The listing builds one solid part. Answer for the finished solid, in the listing's coordinates (mm). Face numbers are marked on the shaded views. A direction names the side the tool comes from. Coordinates: 2 decimals unless noted, no trailing zeros. Order: outer loops, then holes, each group sorted by start corner. A loop starts at its lowest first (then second) coordinate and runs counter-clockwise, first axis right, second up. Notation, with made-up numbers: (75.5, 1) - (112.5, 1) arc R25 ccw to (112.5, 35) - close; hole circle Ø5 at (-12, -5.75). An arc over 180 degrees is marked (long way). Use a Markdown table: item, result. Add a question column.
Item 1: For the marked faces 1 and 2, determine the directions among +Z, -Z, +X, -X, +Y, -Y from which every point of the face is accessible in a straight line to the end or side of a thin tool.
Item 2: The part is cut by section C-C, the plane z = 14.25. State how many separate pieces and enclosed holes the cut face has, then the cut area to 3 significant figures.
Item 3: Flat-ended cylindrical pins translate along their axes: P1, Ø12.5, axis at x = -11, y = 16, coming from the +Z side; P2, Ø12, axis at x = 22.5, y = 22.5, coming from the +Z side. Find the tip coordinate at first contact, or state that the pin passes through.
Item 4: The mould has two halves that part along Y. Classify the marked faces 3, 4, 5 and 6: released by +Y, released by -Y, zero draft, split by the parting line, or undercut.
Item 5: The part is cut by section B-B, the plane y = -19.5. Give the vertices of the cut face in (x, z) (3 decimals), then the cut area to 3 significant figures.
Item 6: The part is cut by section D-D, the plane y = 5. Give the vertices of the cut face in (x, z) (3 decimals), then the cut area to 3 significant figures.
Item 7: The part is cut by section A-A, the plane x = 31.5. Give the vertices of the cut face in (y, z) (3 decimals).
Item 8: Find the intervals of material crossed by line 1 along X through (y, z) = (3, 15.75) (3 decimals); line 2 along Y through (x, z) = (-29.5, 3.25) (3 decimals); line 3 along Y through (x, z) = (-11, 9.5) (3 decimals), in increasing order.
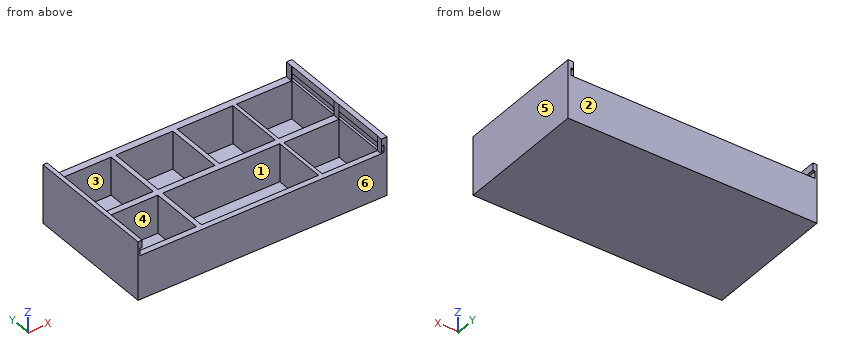
from build123d import *

# Parameters (mm, degrees)
F0_W      = 107.95
F0_H      = 57.15
F1_DEPTH  = 25.4
F2_W      = 25.4
F2_H      = 25.4
F2_H_2    = 23.2541756704
F2_W_2    = 24.6955640614
F2_W_3    = 50.8
F2_H_3    = 23.3953045681
F2_W_4    = 24.2106489923
F2_W_5    = 24.0074023604
F2_H_4    = 23.0993351433
F3_DEPTH  = 22.86
F4_W      = 103.6651358008
F4_H      = 57.15
F5_DEPTH  = 6.35
F6_W      = 57.15
F6_H      = 3.175
F7_DEPTH  = 1.016
F8_W      = 57.15
F8_H      = 3.175
F9_DEPTH  = 1.016
F10_DEPTH = 57.15


with BuildPart() as f1:
    # F0 (on Top) → F1 (new body)
    with BuildSketch(Plane.XY):
        Rectangle(F0_W, F0_H)
    extrude(amount=F1_DEPTH)

    # F2 (on face) → F3 (cut)
    with BuildSketch(Plane.XY.offset(25.4)):
        with Locations((-39.4618835628, 12.7)):
            Rectangle(F2_W, F2_H)
        with Locations((-39.4618835628, -14.386146795)):
            Rectangle(F2_W, F2_H_2)
        with Locations((-12.3477820307, 12.7)):
            Rectangle(F2_W_2, F2_H)
        with Locations((0.7044359386, -14.4567112438)):
            Rectangle(F2_W_3, F2_H_3)
        with Locations((13.9991114425, 12.7)):
            Rectangle(F2_W_4, F2_H)
        with Locations((39.6287105978, 12.7)):
            Rectangle(F2_W_5, F2_H)
        with Locations((39.6287105978, -14.6046959562)):
            Rectangle(F2_W_5, F2_H_4)
    extrude(amount=-F3_DEPTH, mode=Mode.SUBTRACT)

    # F4 (on face) → F5 (cut)
    with BuildSketch(Plane.XY.offset(25.4)):
        with Locations((-0.3293156624, 0)):
            Rectangle(F4_W, F4_H)
    extrude(amount=-F5_DEPTH, mode=Mode.SUBTRACT)

    # F6 (on face) → F7 (cut)
    with BuildSketch(Plane.YZ.offset(-52.1618835628)):
        with Locations((0, 20.6375)):
            Rectangle(F6_W, F6_H)
    extrude(amount=-F7_DEPTH, mode=Mode.SUBTRACT)

    # F8 (on face) → F9 (cut)
    with BuildSketch(Plane(origin=(51.632411778, 0, 0), x_dir=(0, -1, 0), z_dir=(-1, 0, 0))):
        with Locations((0.0344297111, 20.7629382104)):
            Rectangle(F8_W, F8_H)
    extrude(amount=-F9_DEPTH, mode=Mode.SUBTRACT)

    # F10 (cut): a face of the model
    f10_faces = [f1.faces().sort_by_distance(p)[0] for p in [
        (52.140411778, 28.5405702889, 20.7629382104),
    ]]
    extrude(f10_faces, amount=-F10_DEPTH, mode=Mode.SUBTRACT)


solid = f1.part
Solution:
| question | item | result |
|---|---|---|
| 1 | face 1 | +Z |
| 1 | face 2 | +Z, -Z, +X, -X, +Y |
| 2 | separate pieces | 1 |
| 2 | enclosed holes | 7 |
| 2 | area | 1,340 mm2 |
| 3 | P1 | stops at z = 2.54 |
| 3 | P2 | stops at z = 19.05 |
| 4 | face 3 | undercut |
| 4 | face 4 | undercut |
| 4 | face 5 | zero draft |
| 4 | face 6 | released by -Y |
| 5 | outline | (-53.975, 0) - (53.975, 0) - (53.975, 25.4) - (51.632, 25.4) - (51.632, 22.35) - (52.648, 22.35) - (52.648, 19.175) - (51.632, 19.175) - (51.632, 2.54) - (27.625, 2.54) - (27.625, 19.05) - (26.104, 19.05) - (26.104, 2.54) - (-24.696, 2.54) - (-24.696, 19.05) - (-26.762, 19.05) - (-26.762, 2.54) - (-52.162, 2.54) - (-52.162, 19.05) - (-53.178, 19.05) - (-53.178, 22.225) - (-52.162, 22.225) - (-52.162, 25.4) - (-53.975, 25.4) - close |
| 5 | area | 422 mm2 |
| 6 | outline | (-53.975, 0) - (53.975, 0) - (53.975, 25.4) - (51.632, 25.4) - (51.632, 22.35) - (52.648, 22.35) - (52.648, 19.175) - (51.632, 19.175) - (51.632, 2.54) - (27.625, 2.54) - (27.625, 19.05) - (26.104, 19.05) - (26.104, 2.54) - (1.894, 2.54) - (1.894, 19.05) - (0, 19.05) - (0, 2.54) - (-24.696, 2.54) - (-24.696, 19.05) - (-26.762, 19.05) - (-26.762, 2.54) - (-52.162, 2.54) - (-52.162, 19.05) - (-53.178, 19.05) - (-53.178, 22.225) - (-52.162, 22.225) - (-52.162, 25.4) - (-53.975, 25.4) - close |
| 6 | area | 453 mm2 |
| 7 | outline | (-28.575, 0) - (28.575, 0) - (28.575, 19.05) - (25.4, 19.05) - (25.4, 2.54) - (0, 2.54) - (0, 19.05) - (-3.055, 19.05) - (-3.055, 2.54) - (-26.154, 2.54) - (-26.154, 19.05) - (-28.575, 19.05) - close |
| 8 | line 1 | x = -53.975 to -52.162, -26.762 to -24.696, 0 to 1.894, 26.104 to 27.625, 51.632 to 53.975 |
| 8 | line 2 | y = -28.575 to -26.013, -2.759 to 0, 25.4 to 28.575 |
| 8 | line 3 | y = -28.575 to -26.154, -2.759 to 0, 25.4 to 28.575 |
